from build123d import *

# Parameters (mm, degrees)
FLIGHT_COMPUTER_DEPTH = 3


with BuildPart() as part:
    # Sketch2 → Flight Computer (new body)
    with BuildSketch(Plane(origin=(0, 0, 0), x_dir=(1, 0, 0), z_dir=(0, 1, 0))):
        with BuildLine():
            ThreePointArc((-11.25, 12.75), (-12.275658351, 11.326975053), (-13.95, 11.85))
            Line((-13.95, 11.85), (-13.95, -11.85))
            ThreePointArc((-13.95, -11.85), (-12.275658351, -11.326975053), (-11.25, -12.75))
            ThreePointArc((-11.25, -12.75), (-11.408359213, -13.420820393), (-11.85, -13.95))
            Line((-11.85, -13.95), (11.85, -13.95))
            ThreePointArc((11.85, -13.95), (11.689339828, -11.689339828), (13.95, -11.85))
            Line((13.95, -11.85), (13.95, 11.85))
            ThreePointArc((13.95, 11.85), (11.689339828, 11.689339828), (11.85, 13.95))
            Line((11.85, 13.95), (-11.85, 13.95))
            ThreePointArc((-11.85, 13.95), (-11.408359214, 13.420820393), (-11.25, 12.75))
        make_face()
    extrude(amount=FLIGHT_COMPUTER_DEPTH)


solid = part.part
Geometry: final body of the model. Coordinates: model frame, mm. Give positions to 0.01 mm unless a question says otherwise; leave off trailing zeros. Loops run counter-clockwise (first coordinate to the right, second up) from the corner with the lowest first, then second, coordinate; pieces in that order, holes last. Notation, with made-up numbers: (-31, 11) - (6, 11) arc R3 ccw to (6, 16) - close; hole circle Ø8 at (-25, 27). An arc over 180 degrees is marked (long way). Answer as CSV lines item,"result". Start each with the question number.
1. Draft query along X for faces 1 (the face through (13.95, 1, 0)), 2 (the face through (0, 1, 13.95)), 3 (the face through (11.72, 1.48, -11.66)). Return one class per face: released by +X, released by -X, zero draft, split by the parting line, or undercut.
2. Ray query, L1, parallel to X at y = 1.4, z = 12.75. Return the intervals inside material, ascending.
3. Section A-A, the plane y = 0.5. Return loops of the section in (x, z), plus the area to 3 significant figures.
4. Section B-B, the plane x = 12.75. Return loops of the section in (y, z).
Answers:
1,face 1,"released by +X"
1,face 2,"zero draft"
1,face 3,"undercut"
2,L1,"x = -11.25 to 11.25"
3,outline,"(-13.95, -11.85) arc R1.5 cw (long way) to (-11.85, -13.95) - (11.85, -13.95) arc R1.5 cw (long way) to (13.95, -11.85) - (13.95, 11.85) arc R1.5 cw (long way) to (11.85, 13.95) - (-11.85, 13.95) arc R1.5 cw (long way) to (-13.95, 11.85) - close"
3,area,"753 mm2"
4,outline,"(0, -11.25) - (3, -11.25) - (3, 11.25) - (0, 11.25) - close"
